Can you work these out from the drawing? Everything is in mm from the part's minimum corner. A direction names the side the tool comes from. Round coordinates to 2 decimals unless told otherwise and drop trailing zeros. Write each loop counter-clockwise with the first axis right and the second up, starting at its lowest first coordinate (ties: lowest second). Pieces come first, ordered by that corner, then holes. Notation, with made-up numbers: (51, 3) - (102, 3) arc R18 cw to (102, 14) - close; hole circle Ø8 at (32, 29). An arc over 180 degrees is marked (long way). One line per item, written item: value. Start each with the question number.
Item 1: Imagine slicing it at A-A, the plane x = 3.81. Please give me the cut outline in (y, z).
Item 2: For P1, Ø4, axis at x = 4.5, z = 14, coming from the +Y side; P2, Ø2, axis at x = 5.5, z = 9, coming from the -Y side; P3, Ø4, axis at y = 3.5, z = 14.5, coming from the -X side, each with a flat end and sliding along its axis, tell me the tip position at first contact or that it passes through.
Item 3: For the marked faces 1 and 2, which set-ups out of +Z, -Z, +X, -X, +Y, -Y let a thin tool reach every point of the face, with its end or its side?
Item 4: If I drill on line 1 (Z direction, x = 2.75, y = 2.5); line 2 (Z direction, x = 0.75, y = 4.5); line 3 (X direction, y = 4, z = 36.5), over which ranges is the centre line in solid material (lowest first)?
Item 5: Imagine slicing it at C-C, the plane z = 19.5. Please give me the cut outline in (x, y).
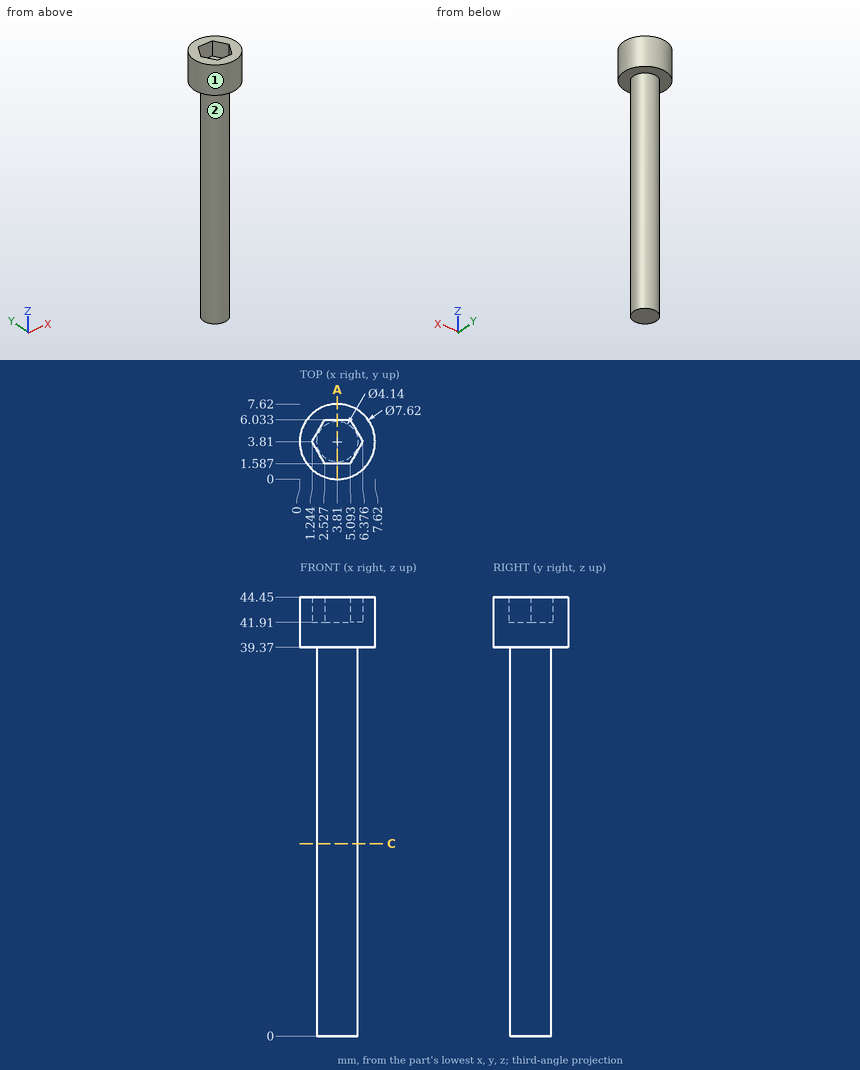
Values follow:
1. outline: (0, 39.37) - (1.74, 39.37) - (1.74, 0) - (5.88, 0) - (5.88, 39.37) - (7.62, 39.37) - (7.62, 44.45) - (6.03, 44.45) - (6.03, 41.91) - (1.59, 41.91) - (1.59, 44.45) - (0, 44.45) - close
2. P1: stops at y = 5.88
2. P2: stops at y = 1.86
2. P3: stops at x = 1.74
3. face 1: +Z, -Z
3. face 2: -Z
4. line 1: z = 0 to 41.91
4. line 2: z = 39.37 to 44.45
4. line 3: x = 1.75 to 5.87
5. outline: circle Ø4.14 at (3.81, 3.81)
